Could you check a few things on this drawing? It's one solid part, dimensions in mm from its lowest x, y, z. A direction names the side the tool comes from. Round coordinates to 2 decimals unless told otherwise and drop trailing zeros. Loops run counter-clockwise (first coordinate to the right, second up) from the corner with the lowest first, then second, coordinate; pieces in that order, holes last. Notation, with made-up numbers: M 12,47 L 36,47 A30 ccw 36,80 Z; hole C -24,-13.75 d2. An arc over 180 degrees is marked long. Use a Markdown table: item, result. Add a question column.
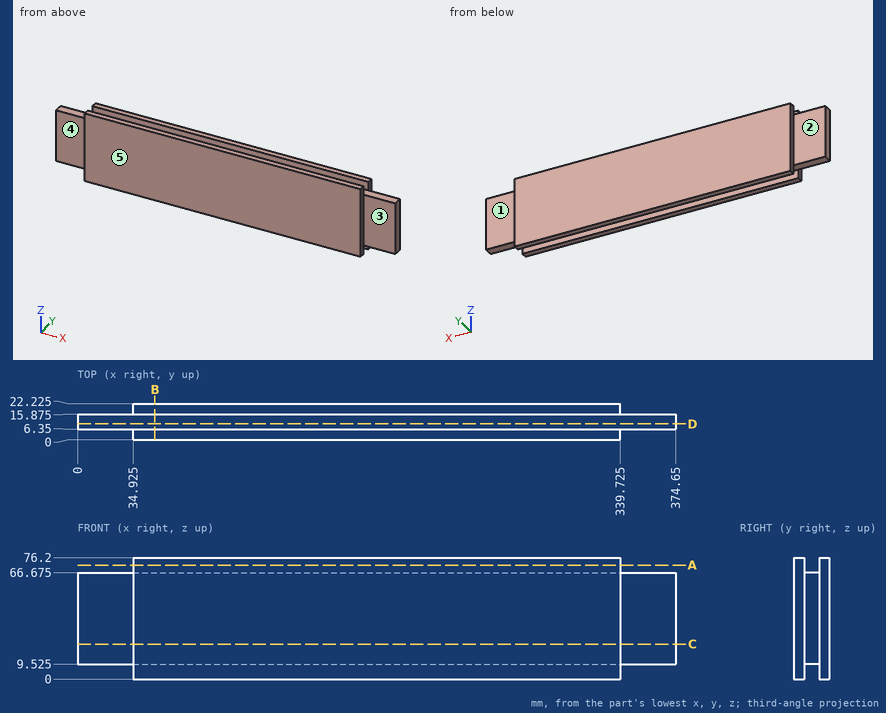
(1) Suppose I cut it at A-A on z = 71.5. List the corners of the cut face in (x, y) for me (3 decimals).
(2) I'm going to push flat-ended pins straight in: pin 1 (3 mm diameter, centred on y = 3.5, z = 50, fed in from -X) (3 decimals); pin 2 (3 mm diameter, centred on x = 193, y = 13.5, fed in from -Z) (3 decimals); pin 3 (7 mm diameter, centred on y = 20, z = 34, fed in from +X) (3 decimals). Where does each tip first touch, or does it pass through?
(3) Suppose I cut it at D-D on y = 9.75. List the corners of the cut face in (x, z) for me (3 decimals).
(4) If I drill on probe 1 along Y at (x, z) = (172.5, 6.5) (3 decimals); probe 2 along X at (y, z) = (2.5, 56.5) (3 decimals); probe 3 along Z at (x, y) = (254, 12.75) (3 decimals), over which ranges is the centre line in solid material (lowest first)? Write a range as [from, to].
(5) Suppose I cut it at C-C on z = 22. List the corners of the cut face in (x, y) for me (3 decimals).
(6) On a 3-axis mill with a long thin cutter (end or side, diameter ignored), from which of +Z, -Z, +X, -X, +Y, -Y can I reach the whole of each face in a straight line? I mean the marked faces 1, 2, 3, 4 and 5. Say none if no direction works.
(7) Suppose I cut it at B-B on x = 48.5. List the corners of the cut face in (y, z) for me (3 decimals).
Results below:
| question | item | result |
|---|---|---|
| 1 | outline | M 34.925,0 L 339.725,0 L 339.725,6.35 L 34.925,6.35 Z; M 34.925,15.875 L 339.725,15.875 L 339.725,22.225 L 34.925,22.225 Z |
| 2 | pin 1 | stops at x = 34.925 |
| 2 | pin 2 | stops at z = 9.525 |
| 2 | pin 3 | stops at x = 339.725 |
| 3 | outline | M 0,9.525 L 374.65,9.525 L 374.65,66.675 L 0,66.675 Z |
| 4 | probe 1 | y = [0, 6.35], [15.875, 22.225] |
| 4 | probe 2 | x = [34.925, 339.725] |
| 4 | probe 3 | z = [9.525, 66.675] |
| 5 | outline | M 0,6.35 L 34.925,6.35 L 34.925,0 L 339.725,0 L 339.725,6.35 L 374.65,6.35 L 374.65,15.875 L 339.725,15.875 L 339.725,22.225 L 34.925,22.225 L 34.925,15.875 L 0,15.875 Z |
| 6 | face 1 | +Z, -Z, +X, +Y |
| 6 | face 2 | +Z, -Z, -X, +Y |
| 6 | face 3 | +Z, -Z, +X, -Y |
| 6 | face 4 | +Z, -Z, -X, -Y |
| 6 | face 5 | +Z, -Z, +X, -X, -Y |
| 7 | outline | M 0,0 L 6.35,0 L 6.35,9.525 L 15.875,9.525 L 15.875,0 L 22.225,0 L 22.225,76.2 L 15.875,76.2 L 15.875,66.675 L 6.35,66.675 L 6.35,76.2 L 0,76.2 Z |
